The model under review builds one solid part; all positions refer to its coordinate system, in mm. A direction names the side the tool comes from. Give positions to 0.01 mm unless a question says otherwise; leave off trailing zeros. Order: outer loops, then holes, each group sorted by start corner. A loop starts at its lowest first (then second) coordinate and runs counter-clockwise, first axis right, second up. Notation, with made-up numbers: (8.25, -15) -> (41.25, -15) arc R25 ccw to (41.25, 8) -> close; hole circle Ø5 at (25.25, 37.25). An arc over 180 degrees is marked (long way). Use one line per item in the form item = value.
Autodesk Inventor part; units mm, degrees
ref_plane "YZ Plane" through (0, 0, 0) normal (1, 0, 0) x (0, 1, 0)
ref_plane "XZ Plane" through (0, 0, 0) normal (0, 1, 0) x (-1, 0, 0)
ref_plane "XY Plane" through (0, 0, 0) normal (0, 0, 1) x (1, 0, 0)
sketch "Sketch1" plane through (0, 0, 0) normal (0, 0, 1) x (1, 0, 0)
  line L0 (0, 0) -> (54.9443, 0)
  line L1 (54.9443, 0) -> (59.3561, 4.4119)
  line L2 (59.3561, 4.4119) -> (59.3561, 59.3561)
  line L3 (59.3561, 59.3561) -> (54.9443, 63.768)
  line L4 (54.9443, 63.768) -> (0, 63.768)
  line L5 (0, 63.768) -> (-4.4114, 59.3566)
  line L6 (-4.4114, 59.3566) -> (-4.4114, 4.4114)
  line L7 (-4.4114, 4.4114) -> (0, 0)
  circle A0 centre (38.6091, 43.0209) radius 2.5
  circle A1 centre (16.3352, 43.0209) radius 2.5
  circle A2 centre (38.6091, 20.7471) radius 2.5
  circle A3 centre (16.3352, 20.7471) radius 2.5
  circle A4 centre (4.9721, 131.884) radius 1.5
  circle A5 centre (49.9721, 131.884) radius 1.5
  line L8 (0, 131.884) -> (0, 141.884)
  line L9 (0, 141.884) -> (54.9443, 141.884)
  line L10 (54.9443, 141.884) -> (54.9443, 131.884)
  line L11 (0, 131.884) -> (0, 121.884)
  line L12 (54.9443, 121.884) -> (54.9443, 131.884)
  line L13 (0, 121.884) -> (4.4114, 117.4726)
  line L14 (50.5324, 117.4721) -> (54.9443, 121.884)
  line L15 (4.4114, 117.4726) -> (4.4114, 63.768)
  line L16 (50.5324, 117.4721) -> (50.5324, 63.768)
  dimension "d3" = 3
  dimension "d4" = 3
  dimension "d5" = 10
  dimension "d6" = 10
extrude "Extrusion1" add sketch "Sketch1" along normal blind 5
chamfer "Chamfer1" distance 5 angle 45 2 edges at (0, 141.884, 2.5) (54.9443, 141.884, 2.5)
sketch "Sketch2" plane through (0, 0, 5) normal (0, 0, 1) x (1, 0, 0)
  line L0 (49.9443, 141.884) -> (54.9443, 136.884)
  line L1 (49.9443, 141.884) -> (5, 141.884)
  line L2 (0, 136.884) -> (5, 141.884)
  line L3 (0, 136.884) -> (0, 121.884)
  line L4 (0, 121.884) -> (4.4114, 117.4726)
  line L5 (4.4114, 117.4726) -> (4.4114, 63.768)
  line L6 (4.4114, 63.768) -> (0, 63.768)
  line L7 (0, 63.768) -> (-4.4114, 59.3566)
  line L8 (-4.4114, 59.3566) -> (-4.4114, 4.4114)
  line L9 (-4.4114, 4.4114) -> (0, 0)
  line L10 (0, 0) -> (54.9443, 0)
  line L11 (54.9443, 0) -> (59.3561, 4.4119)
  line L12 (59.3561, 4.4119) -> (59.3561, 59.3561)
  line L13 (59.3561, 59.3561) -> (54.9443, 63.768)
  line L14 (54.9443, 63.768) -> (50.5324, 63.768)
  line L15 (50.5324, 63.768) -> (50.5324, 117.4721)
  line L16 (50.5324, 117.4721) -> (54.9443, 121.884)
  line L17 (54.9443, 121.884) -> (54.9443, 136.884)
  circle A0 centre (49.9721, 131.884) radius 1.5
  circle A1 centre (4.9721, 131.884) radius 1.5
  circle A2 centre (38.6091, 20.7471) radius 2.5
  circle A3 centre (38.6091, 43.0209) radius 2.5
  circle A4 centre (16.3352, 43.0209) radius 2.5
  circle A5 centre (16.3352, 20.7471) radius 2.5
  circle A6 centre (27.4721, 31.884) radius 9
  dimension "d12" = 18
extrude "Extrusion2" cut sketch "Sketch2" against normal blind 5 contours A6
sketch "Sketch3" plane through (0, 0, 5) normal (0, 0, 1) x (1, 0, 0)
  arc A0 (36.4721, 101.884) -> (18.4721, 101.884) centre (27.4721, 101.884) ccw
  line L0 (18.4721, 101.884) -> (18.4721, 81.884)
  line L1 (36.4721, 101.884) -> (36.4721, 81.884)
  circle A1 centre (27.4721, 31.884) radius 9
  line L2 (27.4721, 71.884) -> (27.4721, 81.884)
  arc A2 (18.4721, 81.884) -> (36.4721, 81.884) centre (27.4721, 81.884) ccw
  point P0 (0, 0)
  dimension "d16" = 18
  dimension "d20" = 10
  dimension "d21" = 18
extrude "Extrusion3" cut sketch "Sketch3" against normal blind 10 contours L1 A2 L0 A0
sketch "Sketch4" plane through (0, 0, 5) normal (0, 0, 1) x (1, 0, 0)
  circle A0 centre (16.3352, 43.0209) radius 2.5
  circle A1 centre (16.3352, 43.0209) radius 2.55
  circle A2 centre (38.6091, 43.0209) radius 2.5
  circle A3 centre (38.6091, 43.0209) radius 2.55
  circle A4 centre (38.6091, 20.7471) radius 2.5
  circle A5 centre (38.6091, 20.7471) radius 2.55
  circle A6 centre (16.3352, 20.7471) radius 2.5
  circle A7 centre (16.3352, 20.7471) radius 2.55
  circle A8 centre (4.9721, 131.884) radius 1.5
  circle A9 centre (4.9721, 131.884) radius 1.55
  circle A10 centre (49.9721, 131.884) radius 1.5
  circle A11 centre (49.9721, 131.884) radius 1.55
  point P0 (0, 0)
  dimension "d22" = 5.1
  dimension "d23" = 5.1
  dimension "d24" = 5.1
  dimension "d25" = 5.1
  dimension "d26" = 3.1
  dimension "d27" = 3.1
extrude "Extrusion4" cut sketch "Sketch4" against normal blind 10 contours A0 | A1 | A2 | A3 | A4 | A5 | A6 | A7 | A8 | A9 | A10 | A11
properties part number "Part1_Camera"
1. Add section B-B on y = 78. Give the boundary of the cut face in (x, z), then the cut area to 3 significant figures.
Values:
outline = (4.41, 0) -> (19.35, 0) -> (19.35, 5) -> (4.41, 5) -> close; (35.59, 0) -> (50.53, 0) -> (50.53, 5) -> (35.59, 5) -> close
area = 149 mm^2
2. The part is to be moulded in two halves that separate along Y. For faces 1 (the face through (27, 72, 5)), 2 (the face through (2.535, 139.419, 2.535)), 3 (the face through (2, 63.768, 2)), 4 (the face through (57.119, 2.175, 2.465)), say which applies: +Y half, -Y half, draft (parallel to the pull), parting line (faces both ways), or undercut.
Values:
face_1 = draft
face_2 = +Y half
face_3 = undercut
face_4 = -Y half
3. Tool access review of faces 5 (the face through (54.944, 129, 2)), 6 (the face through (50.532, 91, 2)), 7 (the face through (27.67, 110.88, 2.54)): name each direction out of +Z, -Z, +X, -X, +Y, -Y from which nothing blocks a thin tool from reaching the whole face with its end or side.
Values:
face_5 = +Z, -Z, +X, +Y
face_6 = +Z, -Z, +X
face_7 = +Z, -Z
4. For L1, parallel to Y at x = 4, z = 2.25; L2, parallel to Y at x = 40, z = 3.05; L3, parallel to X at y = 87, z = 0.8, list the stretches that pass through material, from the lowest coordinate up.
Values:
L1 = 0 to 63.77, 117.88 to 130.68, 133.09 to 140.88
L2 = 0 to 18.61, 22.88 to 40.88, 45.16 to 141.88
L3 = 4.41 to 18.47, 36.47 to 50.53
5. Add section C-C on z = 0.75. Count the separate pieces of the cut face and the enclosed holes in it, then the cut area to 3 significant figures.
Values:
separate_pieces = 1
enclosed_holes = 8
area = 6,840 mm^2
6. For pin 1 Ø6 at (x, y) = (38.61, 43.02) entering from +Z; pin 2 Ø1.5 at (y, z) = (130.5, 3.5) entering from +X; pin 3 Ø1.5 at (y, z) = (131.5, 3) entering from -X; pin 4 Ø2.5 at (y, z) = (96.5, 2) entering from -X, all flat-tipped, find the tip position at first contact; note any pin that passes through.
Values:
pin_1 = 5
pin_2 = 54.94
pin_3 = 0
pin_4 = 4.41
7. Add section A-A on x = 22.5. Give the boundary of the cut face in (y, z).
Values:
outline = (0, 0) -> (24.38, 0) -> (24.38, 5) -> (0, 5) -> close; (39.39, 0) -> (74.38, 0) -> (74.38, 5) -> (39.39, 5) -> close; (109.39, 0) -> (141.88, 0) -> (141.88, 5) -> (109.39, 5) -> close
